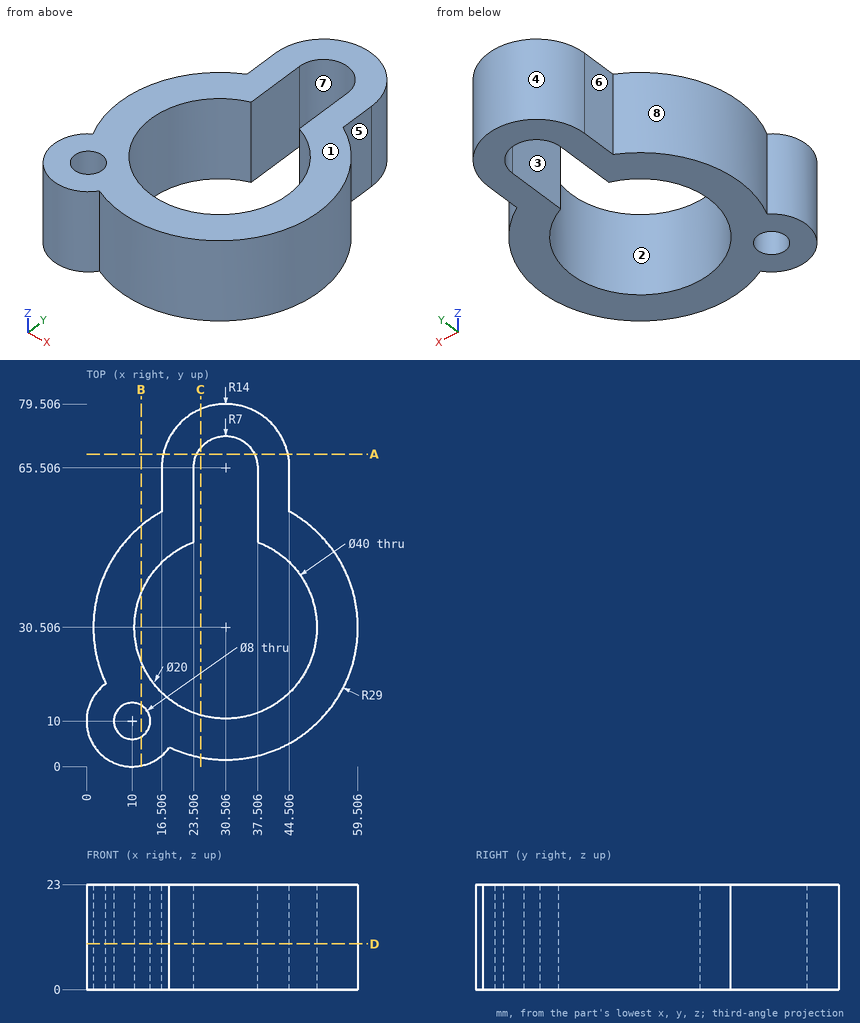
Can you work these out from the drawing? Everything is in mm from the part's minimum corner. A direction names the side the tool comes from. Give positions to 0.01 mm unless a question says otherwise; leave off trailing zeros. Write each loop counter-clockwise with the first axis right and the second up, starting at its lowest first coordinate (ties: lowest second). Pieces come first, ordered by that corner, then holes. Notation, with made-up numbers: M 0.25,59 L 7.25,59 A21 ccw 7.25,69 Z; hole C 25,27 d7. An arc over 180 degrees is marked long. Answer in a Markdown table with one row per item. Add a question column.
Item 1: Please list where these lines run through material, in increasing order: L1, parallel to X at y = 61.5, z = 7.5; L2, parallel to Y at x = 14.5, z = 20.75; L3, parallel to X at y = 69.5, z = 2.75 (1 decimal).
Item 2: Imagine slicing it at B-B, the plane x = 12. Write out the boundary of the cut face in (y, z).
Item 3: We'd pull the mould along Y, two halves only. Please class the marked faces 1, 2, 3 and 4: released by +Y, released by -Y, zero draft, split by the parting line, or undercut.
Item 4: Imagine slicing it at A-A, the plane y = 68.5. Write out the boundary of the cut face in (x, z), plus the area to 3 significant figures.
Item 5: Imagine slicing it at D-D, the plane z = 10. Write out the boundary of the cut face in (x, y), plus the area to 3 significant figures.
Item 6: On a 3-axis mill with a long thin cutter (end or side, diameter ignored), from which of +Z, -Z, +X, -X, +Y, -Y can I reach the whole of each face in a straight line? I mean the marked faces 5, 6, 7 and 8. Say none if no direction works.
Item 7: For pin 1 Ø3 at (x, z) = (40, 12) entering from +Y; pin 2 Ø5 at (y, z) = (61, 16) entering from -X; pin 3 Ø12 at (x, z) = (47.5, 8.5) entering from +Y; pin 4 Ø6 at (x, y) = (16, 37) entering from +Z, each with a flat end and sliding along its axis, tell me the tip position at first contact or that it passes through.
Item 8: Imagine slicing it at C-C, the plane x = 25. Write out the boundary of the cut face in (y, z).
Evaluation:
| question | item | result |
|---|---|---|
| 1 | L1 | x = 16.51 to 23.51, 37.51 to 44.51 |
| 1 | L2 | y = 1.07 to 18.51, 42.5 to 54.69 |
| 1 | L3 | x = 17.1 to 24.8, 36.3 to 43.9 |
| 2 | outline | M 0.2,0 L 6.54,0 L 6.54,23 L 0.2,23 Z; M 13.46,0 L 22.92,0 L 22.92,23 L 13.46,23 Z; M 38.09,0 L 52.83,0 L 52.83,23 L 38.09,23 Z |
| 3 | face 1 | zero draft |
| 3 | face 2 | undercut |
| 3 | face 3 | undercut |
| 3 | face 4 | released by +Y |
| 4 | outline | M 16.83,0 L 24.18,0 L 24.18,23 L 16.83,23 Z; M 36.83,0 L 44.18,0 L 44.18,23 L 36.83,23 Z |
| 4 | area | 338 mm² |
| 5 | outline | M 4.25,18.18 A10 ccw long 18.18,4.25 A29 ccw 44.51,55.9 L 44.51,65.51 A14 ccw 16.51,65.51 L 16.51,55.9 A29 ccw Z; hole C 10,10 d8; hole M 23.51,49.24 A20 ccw long 37.51,49.24 L 37.51,65.51 A7 ccw 23.51,65.51 Z |
| 5 | area | 1,720 mm² |
| 6 | face 5 | +Z, -Z, +X, +Y |
| 6 | face 6 | +Z, -Z, -X, +Y |
| 6 | face 7 | +Z, -Z |
| 6 | face 8 | +Z, -Z, -X |
| 7 | pin 1 | stops at y = 77 |
| 7 | pin 2 | stops at x = 16.51 |
| 7 | pin 3 | stops at y = 74.17 |
| 7 | pin 4 | passes through |
| 8 | outline | M 2.03,0 L 11.28,0 L 11.28,23 L 2.03,23 Z; M 69.83,0 L 78.38,0 L 78.38,23 L 69.83,23 Z |
